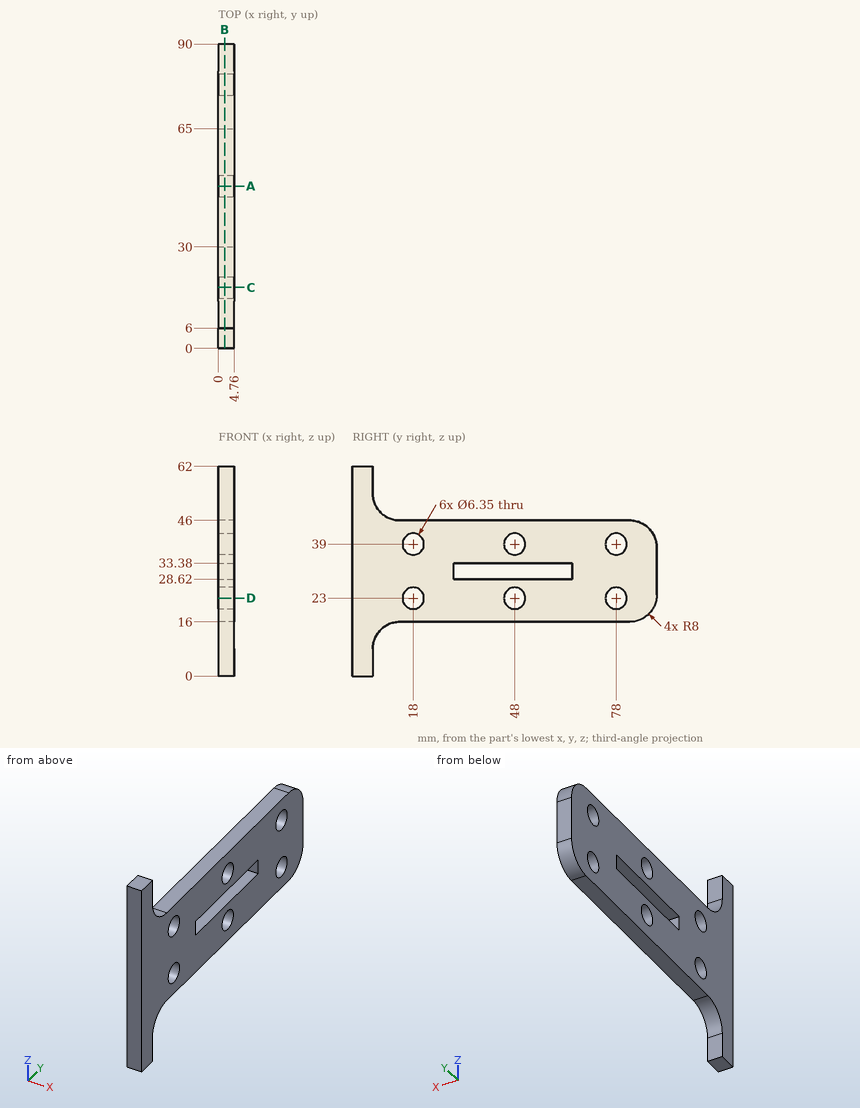
Geometry: see drawing. Coordinates: mm, zero at the bounding-box minimum. Give positions to 0.01 mm unless a question says otherwise; leave off trailing zeros. Order: outer loops, then holes, each group sorted by start corner. A loop starts at its lowest first (then second) coordinate and runs counter-clockwise, first axis right, second up. Notation, with made-up numbers: M -8,-1 L 48,-1 A27 ccw 48,33 Z; hole C 5.5,41 d11. An arc over 180 degrees is marked long. Answer as a JSON object with one key per item and string values.
1. First-contact query: P1, Ø2.5, axis at x = 1.5, z = 3.5, coming from the +Y side; P2, Ø1.4, axis at x = 2, y = 49, coming from the +Z side; P3, Ø2.5, axis at x = 3, y = 45.5, coming from the -Z side. Flat tips, straight axial feed; report the tip coordinate or a pass-through.
Result sheet:
{"P1": "y = 6", "P2": "z = 46", "P3": "z = 16"}
2. Cut plane C-C, the plane y = 18. Output: boundary loops of the cut face in (x, z) (3 decimals), and give its area (3 significant figures).
Result sheet:
{"outline": "M 0,16 L 4.76,16 L 4.76,19.825 L 0,19.825 Z; M 0,26.175 L 4.76,26.175 L 4.76,35.825 L 0,35.825 Z; M 0,42.175 L 4.76,42.175 L 4.76,46 L 0,46 Z", "area": "82.3 mm²"}
3. Cut plane A-A, the plane y = 48. Output: boundary loops of the cut face in (x, z) (3 decimals).
Result sheet:
{"outline": "M 0,16 L 4.76,16 L 4.76,19.825 L 0,19.825 Z; M 0,26.175 L 4.76,26.175 L 4.76,28.62 L 0,28.62 Z; M 0,33.38 L 4.76,33.38 L 4.76,35.825 L 0,35.825 Z; M 0,42.175 L 4.76,42.175 L 4.76,46 L 0,46 Z"}
4. Ray query, line 1 (Y direction, x = 1.1, z = 39) (3 decimals); line 2 (Y direction, x = 3.35, z = 41); line 3 (Z direction, x = 3.85, y = 79.5). Return the intervals inside material, ascending. Write a range as [from, to].
Result sheet:
{"line 1": "[0, 14.825], [21.175, 44.825], [51.175, 74.825], [81.175, 89.937]", "line 2": "[0, 15.53], [20.47, 45.53], [50.47, 75.53], [80.47, 89.42]", "line 3": "[16, 20.2], [25.8, 36.2], [41.8, 46]"}
5. Cut plane D-D, the plane z = 23. Output: boundary loops of the cut face in (x, y) (3 decimals).
Result sheet:
{"outline": "M 0,0 L 4.76,0 L 4.76,14.825 L 0,14.825 Z; M 0,21.175 L 4.76,21.175 L 4.76,44.825 L 0,44.825 Z; M 0,51.175 L 4.76,51.175 L 4.76,74.825 L 0,74.825 Z; M 0,81.175 L 4.76,81.175 L 4.76,89.937 L 0,89.937 Z"}
6. Cut plane B-B, the plane x = 1.9. Output: boundary loops of the cut face in (y, z) (3 decimals), and give its area (3 significant figures).
Result sheet:
{"outline": "M 0,0 L 6,0 L 6,8 A8 cw 14,16 L 82,16 A8 ccw 90,24 L 90,38 A8 ccw 82,46 L 14,46 A8 cw 6,54 L 6,62 L 0,62 Z; hole C 18,23 d6.35; hole C 18,39 d6.35; hole M 30,28.62 L 65,28.62 L 65,33.38 L 30,33.38 Z; hole C 48,23 d6.35; hole C 48,39 d6.35; hole C 78,23 d6.35; hole C 78,39 d6.35", "area": "2,540 mm²"}
